Design review of the part shown in the three views and the two pictorial views. Dimensions are in mm from the part's minimum x, y and z. Coordinates: 2 decimals unless noted, no trailing zeros. Order: outer loops, then holes, each group sorted by start corner. A loop starts at its lowest first (then second) coordinate and runs counter-clockwise, first axis right, second up. Notation, with made-up numbers: (24, 88.25) - (46, 88.25) arc R35 ccw to (46, 124.25) - close; hole circle Ø4 at (83, -24). An arc over 180 degrees is marked (long way). One line per item, written item: value. Start each with the question number.
(1) Consider section C-C on y = 25. Write out the cut boundary in (x, z).
(2) Clearance check with flat-ended pins moving along their axes: pin 1 (3 mm diameter, centred on x = 88, z = 53.5, fed in from -Y) (1 decimal); pin 2 (8 mm diameter, centred on y = 56.5, z = 56.5, fed in from -X); pin 3 (2 mm diameter, centred on x = 42, z = 29, fed in from -Y). State where each tip first meets the part, or that it passes through.
(3) Consider section A-A on z = 19. Write out the cut boundary in (x, y) (1 decimal).
(4) Consider section B-B on x = 66.5. Write out the cut boundary in (y, z) (1 decimal), then the cut area to 3 significant figures.
(5) Consider section D-D on z = 35. Write out the cut boundary in (x, y) (1 decimal).
(6) To check wall thickness, follow line 1 along Z through (x, y) = (63, 59.5); line 2 along X through (y, z) = (28.5, 14) (1 decimal); line 3 along X through (y, z) = (21, 17.5) (1 decimal). State the ranges of each line that lie inside material, in increasing order.
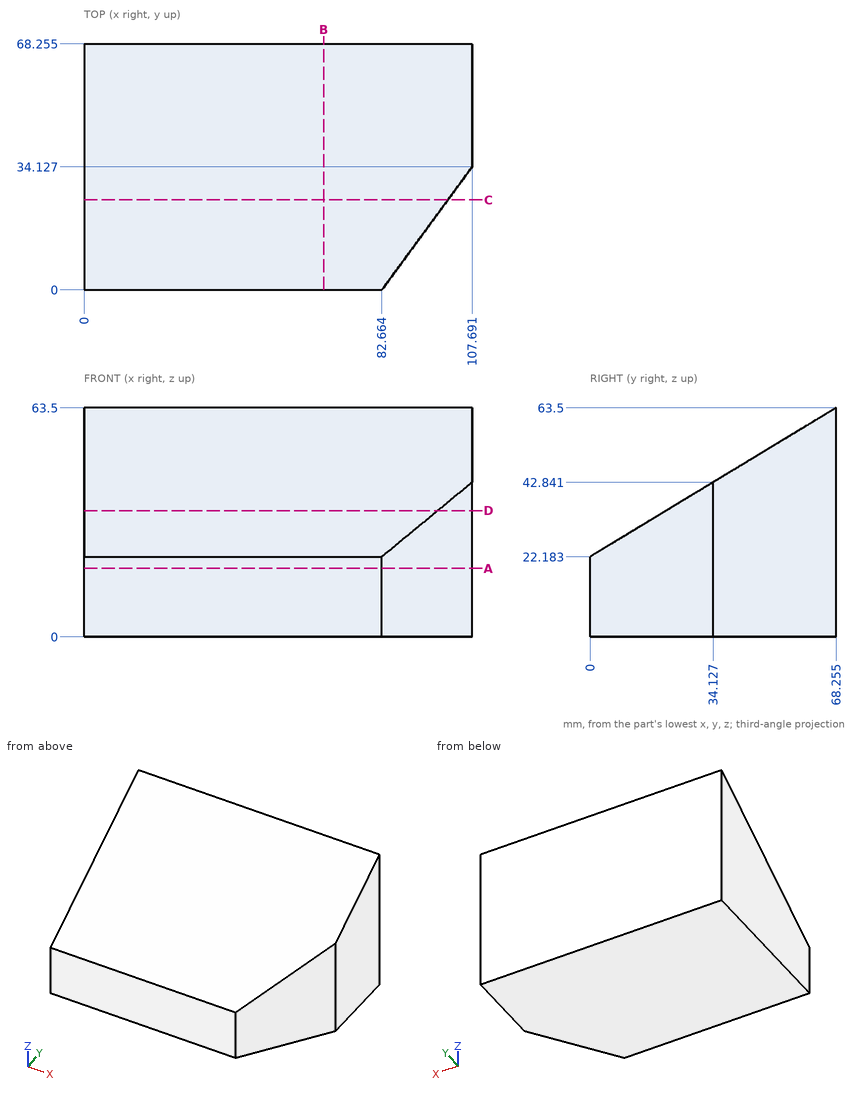
Geometry check:
1. outline: (0, 0) - (101, 0) - (101, 37.32) - (0, 37.32) - close
2. pin 1: stops at y = 49.3
2. pin 2: stops at x = 0
2. pin 3: stops at y = 9.61
3. outline: (0, 0) - (82.7, 0) - (107.7, 34.1) - (107.7, 68.3) - (0, 68.3) - close
4. outline: (0, 0) - (68.3, 0) - (68.3, 63.5) - (0, 22.2) - close
4. area: 2,920 mm^2
5. outline: (0, 21.2) - (98.2, 21.2) - (107.7, 34.1) - (107.7, 68.3) - (0, 68.3) - close
6. line 1: z = 0 to 58.2
6. line 2: x = 0 to 103.6
6. line 3: x = 0 to 98.1
